Geometry: final body of the model. Coordinates: model frame, mm. A direction names the side the tool comes from. Round coordinates to 2 decimals unless told otherwise and drop trailing zeros. Loops run counter-clockwise (first coordinate to the right, second up) from the corner with the lowest first, then second, coordinate; pieces in that order, holes last. Notation, with made-up numbers: (83, 57.5) - (137, 57.5) arc R13 ccw to (137, 65.5) - close; hole circle Ø11 at (4, 61.25). An arc over 180 degrees is marked (long way). Answer as CSV lines item,"result".
from build123d import *

# Parameters (mm, degrees)
CROQUIS1_W              = 98
CROQUIS1_H              = 98
SALIENTE_EXTRUIR1_DEPTH = 9
CHAFL_N1_SIZE2          = 15.588457268
CHAFL_N1_SIZE           = 9
CROQUIS2_W              = 22
CROQUIS2_H              = 35
CORTAR_EXTRUIR1_DEPTH   = 9
CROQUIS3_W              = 15
CROQUIS3_H              = 2.5
SALIENTE_EXTRUIR2_DEPTH = 12.2
CROQUIS4_W              = 15
CROQUIS4_H              = 20.2
SALIENTE_EXTRUIR3_DEPTH = 2.5
CROQUIS5_W              = 5.9
CROQUIS5_H              = 9
CORTAR_EXTRUIR2_DEPTH   = 54.2
CROQUIS6_W              = 15
CROQUIS6_H              = 14.7
SALIENTE_EXTRUIR4_DEPTH = 2.5
SALIENTE_EXTRUIR5_DEPTH = 20
CROQUIS8_W              = 16
CROQUIS8_H              = 15
CORTAR_EXTRUIR3_DEPTH   = 98
CROQUIS9_W              = 16
CROQUIS9_H              = 15
CORTAR_EXTRUIR4_DEPTH   = 13
CROQUIS10_W             = 15
CROQUIS10_H             = 22.7
SALIENTE_EXTRUIR6_DEPTH = 5.3
CROQUIS11_R             = 2
CORTAR_EXTRUIR5_DEPTH   = 10
CROQUIS12_W             = 29.1
CROQUIS12_H             = 5
CORTAR_EXTRUIR6_DEPTH   = 95.963150748
NERVIO1_REACH           = 77.12
CROQUIS13_WALL_W        = 159.310876118
CROQUIS13_WALL_H        = 54
REDONDEO1_R             = 6
CROQUIS14_W             = 15.7
CROQUIS14_H             = 12.7
CORTAR_EXTRUIR7_DEPTH   = 95.963150748


# Some blends are built 0.0001 mm under size
with BuildPart() as part:
    # Croquis1 → Saliente-Extruir1 (new body)
    with BuildSketch(Plane(origin=(0, 0, 0), x_dir=(1, 0, 0), z_dir=(0, 1, 0))):
        Rectangle(CROQUIS1_W, CROQUIS1_H)
    extrude(amount=SALIENTE_EXTRUIR1_DEPTH)

    # Chaflán1
    chafl_n1_edges = [part.edges().sort_by_distance(p)[0] for p in [
        (0, 9, 49),
    ]]
    chafl_n1_side = [part.faces().sort_by_distance(p)[0] for p in [
        (0, 8.82, 49),
    ]]
    chamfer(chafl_n1_edges, length=CHAFL_N1_SIZE - 0.0001, length2=CHAFL_N1_SIZE2 - 0.0001, reference=chafl_n1_side[0])  # a hair under: the kernel refuses the full size

    # Croquis2 → Cortar-Extruir1 (cut)
    with BuildSketch(Plane(origin=(0, 9, 0), x_dir=(1, 0, 0), z_dir=(0, 1, 0))):
        with Locations((-38, 31.5)):
            Rectangle(CROQUIS2_W, CROQUIS2_H)
        with Locations((38, 31.5)):
            Rectangle(CROQUIS2_W, CROQUIS2_H)
    extrude(amount=-CORTAR_EXTRUIR1_DEPTH, mode=Mode.SUBTRACT)

    # Croquis3 → Saliente-Extruir2 (add)
    with BuildSketch(Plane(origin=(0, 9, 0), x_dir=(1, 0, 0), z_dir=(0, 1, 0))):
        with Locations((19.5, 41.85)):
            Rectangle(CROQUIS3_W, CROQUIS3_H)
        with Locations((19.5, 24.15)):
            Rectangle(CROQUIS3_W, CROQUIS3_H)
        with Locations((-19.5, 41.85)):
            Rectangle(CROQUIS3_W, CROQUIS3_H)
        with Locations((-19.5, 24.15)):
            Rectangle(CROQUIS3_W, CROQUIS3_H)
    extrude(amount=SALIENTE_EXTRUIR2_DEPTH)

    # Croquis4 → Saliente-Extruir3 (add)
    with BuildSketch(Plane(origin=(0, 21.2, 0), x_dir=(1, 0, 0), z_dir=(0, 1, 0))):
        with Locations((-19.5, 33)):
            Rectangle(CROQUIS4_W, CROQUIS4_H)
        with Locations((19.5, 33)):
            Rectangle(CROQUIS4_W, CROQUIS4_H)
    extrude(amount=SALIENTE_EXTRUIR3_DEPTH)

    # Croquis5 → Cortar-Extruir2 (cut)
    with BuildSketch(Plane(origin=(27, 0, 0), x_dir=(0, 0, -1), z_dir=(1, 0, 0))):
        with Locations((46.05, 4.5)):
            Rectangle(CROQUIS5_W, CROQUIS5_H)
    extrude(amount=-CORTAR_EXTRUIR2_DEPTH, mode=Mode.SUBTRACT)

    # Croquis6 → Saliente-Extruir4 (add)
    with BuildSketch(Plane.XY.offset(-22.9)):
        with Locations((-19.5, 16.35)):
            Rectangle(CROQUIS6_W, CROQUIS6_H)
        with Locations((19.5, 16.35)):
            Rectangle(CROQUIS6_W, CROQUIS6_H)
    extrude(amount=SALIENTE_EXTRUIR4_DEPTH)

    # Croquis7 → Saliente-Extruir5 (add)
    with BuildSketch(Plane(origin=(0, 9, 0), x_dir=(1, 0, 0), z_dir=(0, 1, 0))):
        Polygon((-49, 14), (-49, -33.411542732), (49, -33.411542732), (49, 14), (36, 14), (36, -20.411542732), (-36, -20.411542732), (-36, 14), align=None)
    extrude(amount=SALIENTE_EXTRUIR5_DEPTH)

    # Croquis8 → Cortar-Extruir3 (cut)
    with BuildSketch(Plane(origin=(49, 0, 0), x_dir=(0, 0, -1), z_dir=(1, 0, 0))):
        with Locations((1, 16.5)):
            Rectangle(CROQUIS8_W, CROQUIS8_H)
    extrude(amount=-CORTAR_EXTRUIR3_DEPTH, mode=Mode.SUBTRACT)

    # Croquis9 → Cortar-Extruir4 (cut)
    with BuildSketch(Plane.XY.offset(33.411542732)):
        with Locations((-28, 16.5)):
            Rectangle(CROQUIS9_W, CROQUIS9_H)
        with Locations((0.5, 16.5)):
            Rectangle(CROQUIS9_W, CROQUIS9_H)
        with Locations((28, 16.5)):
            Rectangle(CROQUIS9_W, CROQUIS9_H)
    extrude(amount=-CORTAR_EXTRUIR4_DEPTH, mode=Mode.SUBTRACT)

    # Croquis10 → Saliente-Extruir6 (add)
    with BuildSketch(Plane(origin=(0, 23.7, 0), x_dir=(1, 0, 0), z_dir=(0, 1, 0))):
        with Locations((-19.5, 31.75)):
            Rectangle(CROQUIS10_W, CROQUIS10_H)
        with Locations((19.5, 31.75)):
            Rectangle(CROQUIS10_W, CROQUIS10_H)
    extrude(amount=SALIENTE_EXTRUIR6_DEPTH)

    # Croquis11 → Cortar-Extruir5 (cut)
    with BuildSketch(Plane(origin=(0, 29, 0), x_dir=(1, 0, 0), z_dir=(0, 1, 0))):
        with Locations(Location((-14, -26.911542732, 0), (0, 0, 270))):
            Circle(CROQUIS11_R)
        with Locations(Location((14, -26.911542732, 0), (0, 0, 270))):
            Circle(CROQUIS11_R)
    extrude(amount=-CORTAR_EXTRUIR5_DEPTH, mode=Mode.SUBTRACT)

    # Croquis12 → Cortar-Extruir6 (cut, through all)
    with BuildSketch(Plane(origin=(27, 0, 0), x_dir=(0, 0, -1), z_dir=(1, 0, 0))):
        with Locations((28.55, 2.5)):
            Rectangle(CROQUIS12_W, CROQUIS12_H)
    extrude(amount=-CORTAR_EXTRUIR6_DEPTH, mode=Mode.SUBTRACT)

    # Croquis13 wall → Nervio1 (add, up to next)
    with BuildSketch(Plane(origin=(0, 2.5, -16.5), x_dir=(0, -0.707106781187, 0.707106781187), z_dir=(0, -0.707106781187, -0.707106781187)), mode=Mode.PRIVATE) as nervio1_sk1:
        Rectangle(CROQUIS13_WALL_W, CROQUIS13_WALL_H)
    nervio1_tool1 = extrude(nervio1_sk1.sketch, amount=-NERVIO1_REACH, mode=Mode.PRIVATE) - part.part
    add(nervio1_tool1.solids().sort_by_distance((0, 2.5, -16.5))[0])

    # Redondeo1
    # the kernel refuses this fillet: 6 mm, written as the material it takes off along each edge
    with BuildSketch(Plane(origin=(42, 5, -43.1), x_dir=(0, 0, 1), z_dir=(-1, 0, 0))) as redondeo1_piece_1:
        with BuildLine():
            CenterArc((REDONDEO1_R, REDONDEO1_R), REDONDEO1_R, 180, 90)
            Line((0, REDONDEO1_R), (0, 0))
            Line((0, 0), (REDONDEO1_R, 0))
        make_face()
    extrude(amount=84, mode=Mode.SUBTRACT)

    # Croquis14 → Cortar-Extruir7 (cut, through all)
    with BuildSketch(Plane(origin=(27, 0, 0), x_dir=(0, 0, -1), z_dir=(1, 0, 0))):
        with Locations((32.75, 15.35)):
            Rectangle(CROQUIS14_W, CROQUIS14_H)
    extrude(amount=-CORTAR_EXTRUIR7_DEPTH, mode=Mode.SUBTRACT)


solid = part.part
(1) Pin query (flat end, axial travel): P1, Ø14, axis at x = 18.5, y = 17, coming from the +Z side; P2, Ø16.5, axis at x = -22.5, z = -34, coming from the -Y side; P3, Ø6, axis at x = -36.5, y = 19, coming from the -Z side. Return the tip coordinate at first contact, or that it passes through.
Findings below:
P1,"z = 33.41"
P2,"y = 5"
P3,"z = -14"
(2) Material intervals for line 1 along X through (y, z) = (15, 26.5); line 2 along Z through (x, y) = (-41, 9.5); line 3 along Y through (x, z) = (-18.5, -31.5), sorted ascending.
Findings below:
line 1,"-49 to -36, -20 to -7.5, 8.5 to 20, 36 to 49"
line 2,"-14 to -9, 7 to 33.41"
line 3,"5 to 9, 21.7 to 29"
(3) Section A-A (z = -5.5). Output: boundary loops of the cut face in (x, y), and give its area (3 significant figures).
Findings below:
outline,"(-49, 0) - (49, 0) - (49, 9) - (-49, 9) - close; (-49, 24) - (-36, 24) - (-36, 29) - (-49, 29) - close; (36, 24) - (49, 24) - (49, 29) - (36, 29) - close"
area,"1,010 mm2"
(4) Draft query along Y for faces 4 (the face through (-0.69, 4.56, 41.1)), 5 (the face through (-20, 19, -20.4)), 6 (the face through (-7.5, 16, 27)). Return one class per face: pulls with the +Y half, pulls with the -Y half, needs draft (parallel to the pull), parting line crosses it, or undercut.
Findings below:
face 4,"pulls with the +Y half"
face 5,"needs draft"
face 6,"undercut"
(5) Access query for faces 1 (the face through (12, 23, -32)), 2 (the face through (-19, 15, -24.9)), 3 (the face through (19, 19, -20.4)). Directions: +Z, -Z, +X, -X, +Y, -Y. A direction counts if a zero-diameter tool reaches every point of the face in a straight line with its end or side. Return the directions, or none.
Findings below:
face 1,"-Z, +Y"
face 2,"+X, -X"
face 3,"+X, -X, +Y"
(6) Section B-B (z = 22.5). Output: boundary loops of the cut face in (x, y), and give its area (3 significant figures).
Findings below:
outline,"(-49, 0) - (49, 0) - (49, 29) - (-49, 29) - close; hole (-36, 9) - (-20, 9) - (-20, 24) - (-36, 24) - close; hole (-7.5, 9) - (8.5, 9) - (8.5, 24) - (-7.5, 24) - close; hole (20, 9) - (36, 9) - (36, 24) - (20, 24) - close"
area,"2,120 mm2"
